Source: three-view drawing plus pictorial views. Frame: mm from the lowest corner of the part. A direction names the side the tool comes from. Coordinates: 2 decimals unless noted, no trailing zeros. Write each loop counter-clockwise with the first axis right and the second up, starting at its lowest first coordinate (ties: lowest second). Pieces come first, ordered by that corner, then holes. Notation, with made-up numbers: (-26.5, -4.75) - (18.5, -4.75) arc R24 ccw to (18.5, 34.25) - close; hole circle Ø5 at (9.25, 55). An arc over 180 degrees is marked (long way). Put each result on its own line as item: value.
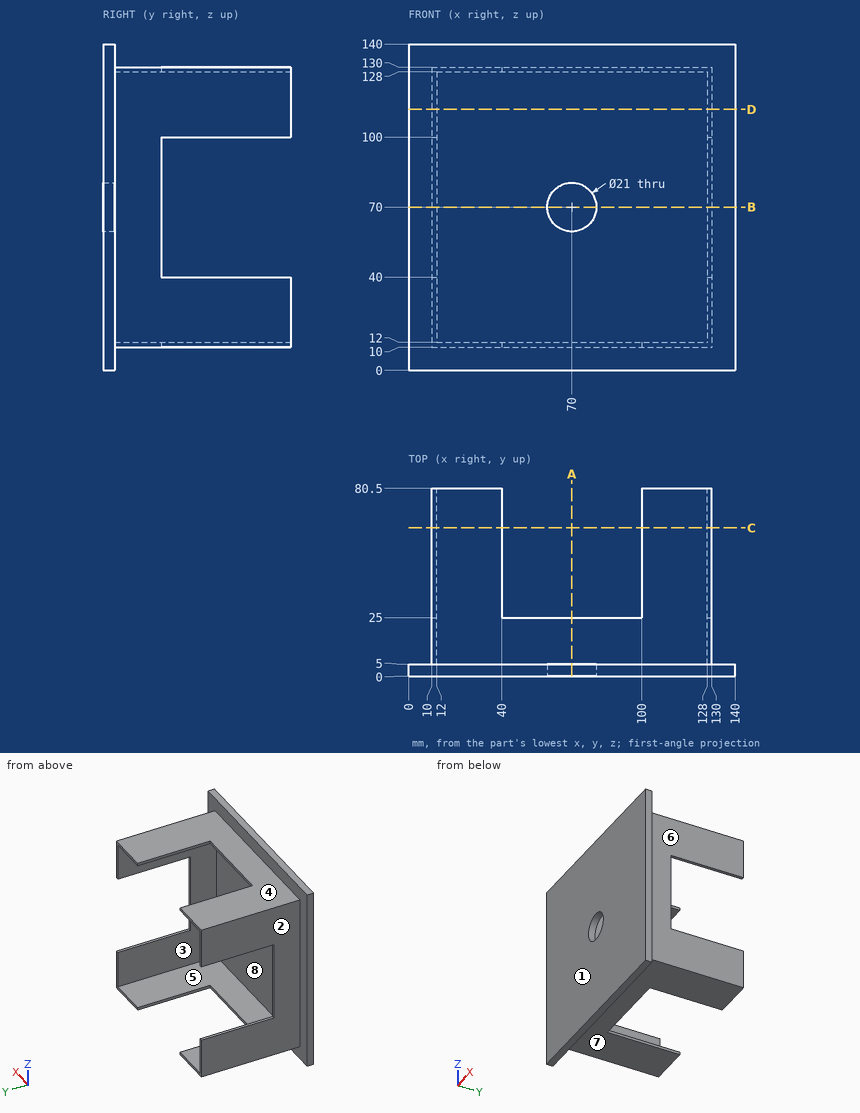
1. Section query A-A (x = 70). Return loops of the section in (y, z).
Answer below:
outline: (0, 0) - (5, 0) - (5, 10) - (25, 10) - (25, 12) - (5, 12) - (5, 59.5) - (0, 59.5) - close; (0, 80.5) - (5, 80.5) - (5, 128) - (25, 128) - (25, 130) - (5, 130) - (5, 140) - (0, 140) - close
2. Section query B-B (z = 70). Return loops of the section in (x, y), then the cut area to 3 significant figures.
Answer below:
outline: (0, 0) - (59.5, 0) - (59.5, 5) - (12, 5) - (12, 25) - (10, 25) - (10, 5) - (0, 5) - close; (80.5, 0) - (140, 0) - (140, 5) - (130, 5) - (130, 25) - (128, 25) - (128, 5) - (80.5, 5) - close
area: 675 mm²
3. Mould query, pull axis X, two halves, no side actions, for the marked faces 5, 6, 7 and 8. Classes: +X half, -X half, draft (parallel to the pull), parting line (faces both ways), or undercut.
Answer below:
face 5: undercut
face 6: +X half
face 7: draft
face 8: undercut
4. Set-up query: the marked faces 1, 2, 3 and 4. Return all of +Z, -Z, +X, -X, +Y, -Y with unobstructed straight access to the full face (end or side cutting, diameter ignored); none if empty.
Answer below:
face 1: +Z, -Z, +X, -X, -Y
face 2: +Z, -Z, -X, +Y
face 3: +Y
face 4: +Z, +X, -X, +Y
5. Section query D-D (z = 112). Return loops of the section in (x, y), then the cut area to 3 significant figures.
Answer below:
outline: (0, 0) - (140, 0) - (140, 5) - (130, 5) - (130, 80.5) - (128, 80.5) - (128, 5) - (12, 5) - (12, 80.5) - (10, 80.5) - (10, 5) - (0, 5) - close
area: 1,000 mm²
6. Ray query, probe 1 along Z at (x, y) = (49, 17.5); probe 2 along X at (y, z) = (2, 70); probe 3 along Y at (x, z) = (134, 90.5). Return the intervals inside material, ascending. Write a range as from..to.
Answer below:
probe 1: z = 10..12, 128..130
probe 2: x = 0..59.5, 80.5..140
probe 3: y = 0..5
7. Section query C-C (y = 63.5). Return loops of the section in (x, z), then the cut area to 3 significant figures.
Answer below:
outline: (10, 10) - (40, 10) - (40, 12) - (12, 12) - (12, 40) - (10, 40) - close; (10, 100) - (12, 100) - (12, 128) - (40, 128) - (40, 130) - (10, 130) - close; (100, 10) - (130, 10) - (130, 40) - (128, 40) - (128, 12) - (100, 12) - close; (100, 128) - (128, 128) - (128, 100) - (130, 100) - (130, 130) - (100, 130) - close
area: 464 mm²
8. Pin query (flat end, axial travel): pin 1 Ø1 at (x, y) = (11.5, 49.5) entering from +Z; pin 2 Ø8 at (x, z) = (107.5, 24) entering from +Y; pin 3 Ø22.5 at (y, z) = (57, 92) entering from -X. Return the tip coordinate at first contact, or that it passes through.
Answer below:
pin 1: stops at z = 130
pin 2: stops at y = 5
pin 3: stops at x = 10
